```python
from build123d import *

# Parameters (mm, degrees)
ESQUISSE1_W        = 60
ESQUISSE1_H        = 60
ESQUISSE1_R        = 6
ESQUISSE1_R_2      = 1
BOSS_EXTRU_1_DEPTH = 2
ESQUISSE2_R        = 10
ESQUISSE2_R_2      = 8.25
BOSS_EXTRU_2_DEPTH = 50
CONG_1_R           = 5


with BuildPart() as part:
    # Esquisse1 → Boss.-Extru.1 (new body)
    with BuildSketch(Plane.XY):
        Rectangle(ESQUISSE1_W, ESQUISSE1_H)
        Circle(ESQUISSE1_R, mode=Mode.SUBTRACT)
        with Locations((-26, 26)):
            Circle(ESQUISSE1_R_2, mode=Mode.SUBTRACT)
        with Locations((26, 26)):
            Circle(ESQUISSE1_R_2, mode=Mode.SUBTRACT)
        with Locations((26, -26)):
            Circle(ESQUISSE1_R_2, mode=Mode.SUBTRACT)
        with Locations((-26, -26)):
            Circle(ESQUISSE1_R_2, mode=Mode.SUBTRACT)
    extrude(amount=BOSS_EXTRU_1_DEPTH)

    # Esquisse2 → Boss.-Extru.2 (add)
    with BuildSketch(Plane.XY.offset(2)):
        Circle(ESQUISSE2_R)
        Circle(ESQUISSE2_R_2, mode=Mode.SUBTRACT)
    extrude(amount=BOSS_EXTRU_2_DEPTH)

    # Congé1
    cong_1_edges = [part.edges().sort_by_distance(p)[0] for p in [
        (-10, 0, 2),
    ]]
    fillet(cong_1_edges, radius=CONG_1_R)


solid = part.part
```
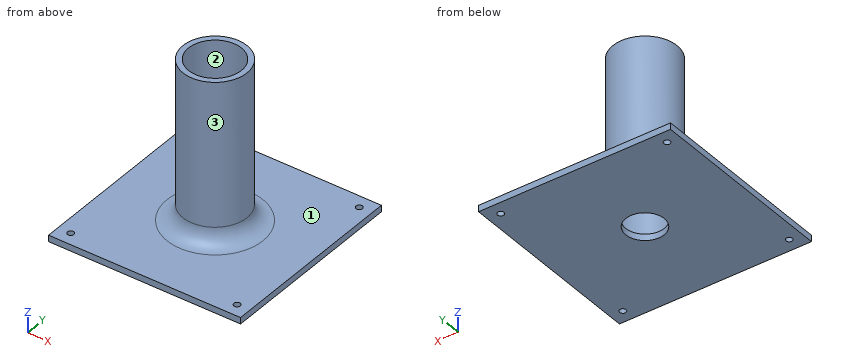
The listing builds one solid part. Answer for the finished solid, in the listing's coordinates (mm). Face numbers are marked on the shaded views. Round coordinates to 2 decimals unless told otherwise and drop trailing zeros. Loops run counter-clockwise (first coordinate to the right, second up) from the corner with the lowest first, then second, coordinate; pieces in that order, holes last.
Q1. Section B-B, the plane y = 26 is taken. Determine the outline of the cut face in (x, z).
Q2. Section A-A, the plane y = 0 is taken. Determine the outline of the cut face in (x, z).
Q3. For a pull along Y with two mould halves and no side action, classify the marked faces 1, 2 and 3 as released by +Y, released by -Y, zero draft, split by the parting line, or undercut.
Q4. Find the intervals of material crossed by line 1 (Y direction, x = 26, z = 1); line 2 (Y direction, x = 0, z = 0.5); line 3 (Z direction, x = -24.5, y = 3.5), in increasing order.
Q5. Section D-D, the plane z = 25 is taken. Determine the outline of the cut face in (x, y).
Q6. Given pin 1 Ø1 at (x, z) = (-8, 41) entering from +Y; pin 2 Ø6 at (y, z) = (-3, 13) entering from +X; pin 3 Ø14 at (x, y) = (0, 0) entering from +Z, each flat-ended and moving along its own axis, determine where each tip first touches the part or whether it passes through.
Completed:
1. outline: (-30, 0) - (-27, 0) - (-27, 2) - (-30, 2) - close; (-25, 0) - (25, 0) - (25, 2) - (-25, 2) - close; (27, 0) - (30, 0) - (30, 2) - (27, 2) - close
2. outline: (-30, 0) - (-6, 0) - (-6, 2) - (-8.25, 2) - (-8.25, 52) - (-10, 52) - (-10, 7) arc R5 cw to (-15, 2) - (-30, 2) - close; (6, 0) - (30, 0) - (30, 2) - (15, 2) arc R5 cw to (10, 7) - (10, 52) - (8.25, 52) - (8.25, 2) - (6, 2) - close
3. face 1: zero draft
3. face 2: undercut
3. face 3: split by the parting line
4. line 1: y = -30 to -27, -25 to 25, 27 to 30
4. line 2: y = -30 to -6, 6 to 30
4. line 3: z = 0 to 2
5. outline: circle Ø20 at (0, 0); hole circle Ø16.5 at (0, 0)
6. pin 1: stops at y = 6.61
6. pin 2: stops at x = 10
6. pin 3: stops at z = 2
